```python
from build123d import *

# Parameters (mm, degrees)
SKETCH2_R           = 11
BOSS_EXTRUDE1_DEPTH = 7.2
SKETCH3_R           = 4.15
SKETCH3_R_2         = 1.25
CUT_EXTRUDE1_DEPTH  = 8.2


with BuildPart() as part:
    # Sketch2 → Boss-Extrude1 (new body)
    with BuildSketch(Plane.XY):
        Circle(SKETCH2_R)
    extrude(amount=BOSS_EXTRUDE1_DEPTH)

    # Sketch3 → Cut-Extrude1 (cut, through all)
    with BuildSketch(Plane(origin=(0, 0, 0), x_dir=(-1, 0, 0), z_dir=(0, 0, -1))):
        Circle(SKETCH3_R)
        with Locations((8, 0)):
            Circle(SKETCH3_R_2)
        with Locations((5.656854249, -5.656854249)):
            Circle(SKETCH3_R_2)
        with Locations((0, -8)):
            Circle(SKETCH3_R_2)
        with Locations((-5.656854249, -5.656854249)):
            Circle(SKETCH3_R_2)
        with Locations((-8, 0)):
            Circle(SKETCH3_R_2)
        with Locations((-5.656854249, 5.656854249)):
            Circle(SKETCH3_R_2)
        with Locations((0, 8)):
            Circle(SKETCH3_R_2)
        with Locations((5.656854249, 5.656854249)):
            Circle(SKETCH3_R_2)
    extrude(amount=-CUT_EXTRUDE1_DEPTH, mode=Mode.SUBTRACT)


solid = part.part
```
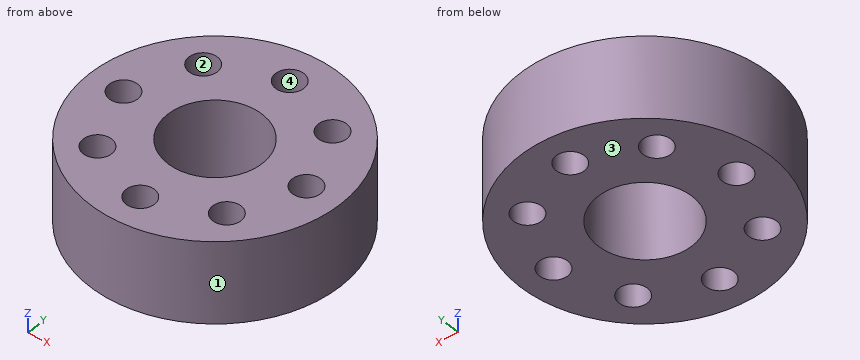
Source: CAD feature listing. Evaluate the final solid. Frame: model axes, mm. Face numbers are marked on the shaded views. Coordinates: 2 decimals unless noted, no trailing zeros. Loops run counter-clockwise (first coordinate to the right, second up) from the corner with the lowest first, then second, coordinate; pieces in that order, holes last. Notation, with made-up numbers: M -31.5,9 L -14.5,9 A11 cw -14.5,16 Z; hole C -30,63.5 d3. An arc over 180 degrees is marked long. Put each result on its own line as item: value. Start each with the question number.
1) Contact query for flat-ended pins moving along their axis: pin 1 Ø4 at (x, y) = (5.66, -5.66) entering from -Z; pin 2 Ø1.5 at (x, y) = (-5.66, -5.66) entering from +Z; pin 3 Ø1 at (y, z) = (5.5, 3.5) entering from +X; pin 4 Ø1.5 at (x, z) = (-5, 5) entering from -Y. Output: stop coordinate, or through.
2) Cut plane A-A on y = 0. Return the cut outline in (x, z), then the cut area to 3 significant figures.
3) Pull-direction query (Y, two-part tool) for the marked faces 1, 2, 3 and 4; classes: pulls with the +Y half, pulls with the -Y half, needs draft (parallel to the pull), parting line crosses it, or undercut.
4) Ray query, L1, parallel to X at y = 0.25, z = 3; L2, parallel to Y at x = 0.5, z = 3.75; L3, parallel to X at y = 5.5, z = 1.75. Return the intervals inside material, ascending. Write a range as from..to.
5) Cut plane D-D on x = 6. Return the cut outline in (y, z).
6) Cut plane C-C on x = 2.5. Return the cut outline in (y, z).
The answers:
1. pin 1: stops at z = 0
1. pin 2: passes through
1. pin 3: stops at x = 9.8
1. pin 4: stops at y = -10.15
2. outline: M -11,0 L -9.25,0 L -9.25,7.2 L -11,7.2 Z; M -6.75,0 L -4.15,0 L -4.15,7.2 L -6.75,7.2 Z; M 4.15,0 L 6.75,0 L 6.75,7.2 L 4.15,7.2 Z; M 9.25,0 L 11,0 L 11,7.2 L 9.25,7.2 Z
2. area: 62.6 mm²
3. face 1: parting line crosses it
3. face 2: undercut
3. face 3: needs draft
3. face 4: undercut
4. L1: x = -11..-9.22, -6.78..-4.14, 4.14..6.78, 9.22..11
4. L2: y = -10.99..-9.15, -6.85..-4.12, 4.12..6.85, 9.15..10.99
4. L3: x = -9.53..-6.9, -4.42..4.42, 6.9..9.53
5. outline: M -9.22,0 L -6.86,0 L -6.86,7.2 L -9.22,7.2 Z; M -4.45,0 L 4.45,0 L 4.45,7.2 L -4.45,7.2 Z; M 6.86,0 L 9.22,0 L 9.22,7.2 L 6.86,7.2 Z
6. outline: M -10.71,0 L -3.31,0 L -3.31,7.2 L -10.71,7.2 Z; M 3.31,0 L 10.71,0 L 10.71,7.2 L 3.31,7.2 Z
